Verification items for the finished model (mm, model axes). Round coordinates to 2 decimals unless told otherwise and drop trailing zeros. Write each loop counter-clockwise with the first axis right and the second up, starting at its lowest first coordinate (ties: lowest second). Pieces come first, ordered by that corner, then holes. Notation, with made-up numbers: M 13,35.25 L 28,35.25 A18 ccw 28,44.25 Z; hole C -0.5,46.25 d1. An arc over 180 degrees is marked long. One line per item, written item: value. Start each with the question number.
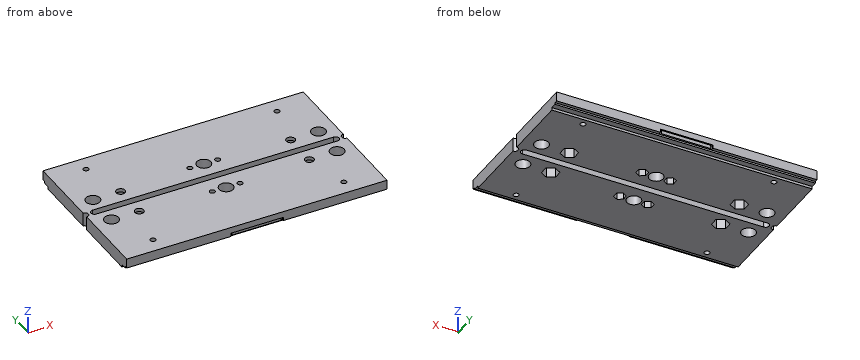
from build123d import *

# Parameters (mm, degrees)
SKETCH_2_W           = 150
SKETCH_2_H           = 43
SKETCH_2_R           = 4.05
EXTRUDE_1_DEPTH      = 8
SKETCH_3_R           = 2.55
CUT_EXTRUDE_1_DEPTH  = 157.246599963
CUT_EXTRUDE_16_DEPTH = 6
CUT_EXTRUDE_2_DEPTH  = 157.246599963
SKETCH_5_R           = 1.55
CUT_EXTRUDE_3_DEPTH  = 157.246599963
CUT_EXTRUDE_5_DEPTH  = 4.5
SKETCH_25_R          = 1.55
CUT_EXTRUDE_13_DEPTH = 157.246599963
CUT_EXTRUDE_11_DEPTH = 2
EXTRUDE_2_DEPTH      = 8


with BuildPart() as part:
    # 草图2 → 凸台-拉伸1 (new body)
    with BuildSketch(Plane.XY):
        with Locations((75, 21.5)):
            Rectangle(SKETCH_2_W, SKETCH_2_H)
        with Locations((10, 8)):
            Circle(SKETCH_2_R, mode=Mode.SUBTRACT)
        with Locations((75, 10)):
            Circle(SKETCH_2_R, mode=Mode.SUBTRACT)
        with Locations((140, 8)):
            Circle(SKETCH_2_R, mode=Mode.SUBTRACT)
    extrude_1 = extrude(amount=EXTRUDE_1_DEPTH)

    # 草图3 → 切除-拉伸1 (cut, through all)
    with BuildSketch(Plane.XY.offset(8)):
        with Locations((26, 8)):
            Circle(SKETCH_3_R)
        with Locations((124, 8)):
            Circle(SKETCH_3_R)
    cut_extrude_1 = extrude(amount=-CUT_EXTRUDE_1_DEPTH, mode=Mode.SUBTRACT)

    # 草图28 → 切除-拉伸16 (cut)
    with BuildSketch(Plane(origin=(0, 0, 0), x_dir=(-1, 0, 0), z_dir=(0, 0, -1))):
        Polygon((-119.9, 5.632863896), (-119.9, 10.367136104), (-124, 12.734272207), (-128.1, 10.367136104), (-128.1, 5.632863896), (-124, 3.265727793), align=None)
        Polygon((-21.9, 5.632863896), (-21.9, 10.367136104), (-26, 12.734272207), (-30.1, 10.367136104), (-30.1, 5.632863896), (-26, 3.265727793), align=None)
    cut_extrude_16 = extrude(amount=-CUT_EXTRUDE_16_DEPTH, mode=Mode.SUBTRACT)

    # 草图4 → 切除-拉伸2 (cut, through all)
    with BuildSketch(Plane(origin=(150, 0, 0), x_dir=(0, 0, -1), z_dir=(1, 0, 0))):
        Polygon((-1.5, 41.2), (-2.5, 41.2), (-2.5, 43), (0, 43), (0, 37.8), (-1.5, 37.8), align=None)
    cut_extrude_2 = extrude(amount=-CUT_EXTRUDE_2_DEPTH, mode=Mode.SUBTRACT)

    # 草图5 → 切除-拉伸3 (cut, through all)
    with BuildSketch(Plane.XY.offset(8)):
        with Locations((83, 10)):
            Circle(SKETCH_5_R)
        with Locations((67, 10)):
            Circle(SKETCH_5_R)
    cut_extrude_3 = extrude(amount=-CUT_EXTRUDE_3_DEPTH, mode=Mode.SUBTRACT)

    # 草图8 → 切除-拉伸5 (cut)
    with BuildSketch(Plane(origin=(0, 0, 0), x_dir=(-1, 0, 0), z_dir=(0, 0, -1))):
        Polygon((-80.15, 8.354551733), (-80.15, 11.645448267), (-83, 13.290896534), (-85.85, 11.645448267), (-85.85, 8.354551733), (-83, 6.709103466), align=None)
        Polygon((-64.15, 8.354551733), (-64.15, 11.645448267), (-67, 13.290896534), (-69.85, 11.645448267), (-69.85, 8.354551733), (-67, 6.709103466), align=None)
    cut_extrude_5 = extrude(amount=-CUT_EXTRUDE_5_DEPTH, mode=Mode.SUBTRACT)

    # 草图25 → 切除-拉伸13 (cut, through all)
    with BuildSketch(Plane(origin=(0, 0, 0), x_dir=(-1, 0, 0), z_dir=(0, 0, -1))):
        with Locations((-130, 34)):
            Circle(SKETCH_25_R)
        with Locations((-20, 34)):
            Circle(SKETCH_25_R)
    cut_extrude_13 = extrude(amount=-CUT_EXTRUDE_13_DEPTH, mode=Mode.SUBTRACT)

    # 草图19 → 切除-拉伸11 (cut)
    with BuildSketch(Plane(origin=(0, 0, 2.5), x_dir=(-1, 0, 0), z_dir=(0, 0, -1))):
        with BuildLine():
            Line((-60, 43), (-90.247938178, 43))
            Line((-90.247938178, 43), (-90.247938178, 42.2))
            ThreePointArc((-90.247938178, 42.2), (-89.747938178, 41.7), (-89.247938178, 42.2))
            Line((-89.247938178, 42.2), (-61, 42.2))
            ThreePointArc((-61, 42.2), (-60.5, 41.7), (-60, 42.2))
            Line((-60, 42.2), (-60, 43))
        make_face()
    cut_extrude_11 = extrude(amount=-CUT_EXTRUDE_11_DEPTH, mode=Mode.SUBTRACT)

    # 草图22 → 凸台-拉伸2 (add)
    with BuildSketch(Plane.XY.offset(8)):
        with BuildLine():
            Line((0, -4), (5.5, -4))
            ThreePointArc((5.5, -4), (3.5, -2), (5.5, 0))
            Line((5.5, 0), (0, 0))
            ThreePointArc((0, 0), (2, -2), (0, -4))
        make_face()
        with BuildLine():
            Line((150, 0), (144.5, 0))
            ThreePointArc((144.5, 0), (146.5, -2), (144.5, -4))
            Line((144.5, -4), (150, -4))
            ThreePointArc((150, -4), (148, -2), (150, 0))
        make_face()
    extrude(amount=-EXTRUDE_2_DEPTH)

    # 镜向2: 凸台-拉伸1, 切除-拉伸1, 切除-拉伸16, 切除-拉伸2, 切除-拉伸3, 切除-拉伸5, 切除-拉伸13, 切除-拉伸11 across plane
    add(extrude_1.mirror(Plane(origin=(0, -2, 0), x_dir=(0, 0, 1), z_dir=(0, -1, 0))))
    add(cut_extrude_1.mirror(Plane(origin=(0, -2, 0), x_dir=(0, 0, 1), z_dir=(0, -1, 0))), mode=Mode.SUBTRACT)
    add(cut_extrude_16.mirror(Plane(origin=(0, -2, 0), x_dir=(0, 0, 1), z_dir=(0, -1, 0))), mode=Mode.SUBTRACT)
    add(cut_extrude_2.mirror(Plane(origin=(0, -2, 0), x_dir=(0, 0, 1), z_dir=(0, -1, 0))), mode=Mode.SUBTRACT)
    add(cut_extrude_3.mirror(Plane(origin=(0, -2, 0), x_dir=(0, 0, 1), z_dir=(0, -1, 0))), mode=Mode.SUBTRACT)
    add(cut_extrude_5.mirror(Plane(origin=(0, -2, 0), x_dir=(0, 0, 1), z_dir=(0, -1, 0))), mode=Mode.SUBTRACT)
    add(cut_extrude_13.mirror(Plane(origin=(0, -2, 0), x_dir=(0, 0, 1), z_dir=(0, -1, 0))), mode=Mode.SUBTRACT)
    add(cut_extrude_11.mirror(Plane(origin=(0, -2, 0), x_dir=(0, 0, 1), z_dir=(0, -1, 0))), mode=Mode.SUBTRACT)


solid = part.part
1) Thickness scan on line 1 (Y direction, x = 67, z = 5.6); line 2 (Y direction, x = 140, z = 4); line 3 (X direction, y = -2, z = 3.75). Record the ranges inside material, lowest first.
2) Cross-section at B-B (y = 34). Record the boundary of the cut face in (x, z), then the cut area to 3 significant figures.
3) Gauge pin test, flat ends, axial feed: pin 1 Ø6.5 at (x, y) = (125, -10.5) entering from -Z; pin 2 Ø1 at (x, z) = (69.5, 3) entering from -Y; pin 3 Ø0.5 at (x, y) = (104.5, 42) entering from -Z. Record the tip position at first contact, or that the pin passes through.
4) Cross-section at A-A (x = 10). Record the boundary of the cut face in (y, z).
5) Cross-section at D-D (y = -2.5). Record the boundary of the cut face in (x, z), then the cut area to 3 significant figures.
6) Cross-section at C-C (x = 113.5). Record the boundary of the cut face in (y, z).
Results below:
1. line 1: y = -47 to -15.55, -12.45 to -4, 0 to 8.45, 11.55 to 43
1. line 2: y = -47 to -16.05, -7.95 to -4, 0 to 3.95, 12.05 to 43
1. line 3: x = 2 to 3.5, 146.5 to 148
2. outline: M 0,0 L 18.45,0 L 18.45,8 L 0,8 Z; M 21.55,0 L 128.45,0 L 128.45,8 L 21.55,8 Z; M 131.55,0 L 150,0 L 150,8 L 131.55,8 Z
2. area: 1,150 mm²
3. pin 1: stops at z = 0
3. pin 2: stops at y = -46.2
3. pin 3: stops at z = 2.5
4. outline: M -47,2.5 L -45.2,2.5 L -45.2,1.5 L -41.8,1.5 L -41.8,0 L -16.05,0 L -16.05,8 L -47,8 Z; M -7.95,0 L -4,0 L -4,8 L -7.95,8 Z; M 0,0 L 3.95,0 L 3.95,8 L 0,8 Z; M 12.05,0 L 37.8,0 L 37.8,1.5 L 41.2,1.5 L 41.2,2.5 L 43,2.5 L 43,8 L 12.05,8 Z
5. outline: M 1.94,0 L 3.56,0 L 3.56,8 L 1.94,8 Z; M 146.44,0 L 148.06,0 L 148.06,8 L 146.44,8 Z
5. area: 26.0 mm²
6. outline: M -47,2.5 L -45.2,2.5 L -45.2,1.5 L -41.8,1.5 L -41.8,0 L -4,0 L -4,8 L -47,8 Z; M 0,0 L 37.8,0 L 37.8,1.5 L 41.2,1.5 L 41.2,2.5 L 43,2.5 L 43,8 L 0,8 Z
